```python
from build123d import *

# Parameters (mm, degrees)
SKETCH_5_R          = 36
CUT_EXTRUDE_1_DEPTH = 191
SKETCH_6_R          = 3
CUT_EXTRUDE_3_DEPTH = 225
SKETCH_7_R          = 2.7
CUT_EXTRUDE_4_DEPTH = 111


with BuildPart() as part:
    # 草图1 → 旋转6 (revolve)
    with BuildSketch(Plane(origin=(0, 0, 0), x_dir=(0, 0, -1), z_dir=(1, 0, 0)), mode=Mode.PRIVATE) as revolve_6_sk:
        with BuildLine():
            Line((3.317174788, 159.625816033), (43.317174788, 159.625816033))
            Line((43.317174788, 159.625816033), (73.317174788, 159.625816033))
            Line((73.317174788, 159.625816033), (73.317174788, 179.625816033))
            Line((73.317174788, 179.625816033), (81.317174788, 179.625816033))
            Line((81.317174788, 179.625816033), (81.317174788, 154.625816033))
            Line((81.317174788, 154.625816033), (73.317174788, 154.625816033))
            Line((73.317174788, 154.625816033), (53.317174788, 154.625816033))
            Line((53.317174788, 154.625816033), (53.317174788, 94.625816033))
            Line((53.317174788, 94.625816033), (43.317174788, 94.625816033))
            Line((43.317174788, 94.625816033), (43.317174788, 154.625816033))
            Line((43.317174788, 154.625816033), (3.317174788, 154.625816033))
            ThreePointArc((3.317174788, 154.625816033), (-39.109232083, 137.052222904), (-56.682825212, 94.625816033))
            Line((-56.682825212, 94.625816033), (-61.682825212, 94.625816033))
            ThreePointArc((-61.682825212, 94.625816033), (-42.644765989, 140.58775681), (3.317174788, 159.625816033))
        make_face()
    revolve(revolve_6_sk.sketch.rotate(Axis((0, 94.625816033, -43.317174788), (0, 0, -1)), 90), axis=Axis((0, 94.625816033, -43.317174788), (0, 0, -1)))

    # 草图5 → 切除-拉伸1 (cut)
    with BuildSketch(Plane(origin=(0, 0, 0), x_dir=(1, 0, 0), z_dir=(0, 1, 0))):
        with Locations(Location((0, 5.317174788, 0), (0, 0, 183.184738537))):
            Circle(SKETCH_5_R)
    extrude(amount=CUT_EXTRUDE_1_DEPTH, mode=Mode.SUBTRACT)

    # 草图6 → 切除-拉伸3 (cut)
    with BuildSketch(Plane.XY):
        with Locations((0, 169.625816033)):
            Circle(SKETCH_6_R)
        with Locations((0, 19.625816033)):
            Circle(SKETCH_6_R)
        with Locations((64.951905284, 132.125816033)):
            Circle(SKETCH_6_R)
        with Locations((64.951905284, 57.125816033)):
            Circle(SKETCH_6_R)
        with Locations((-64.951905284, 132.125816033)):
            Circle(SKETCH_6_R)
        with Locations((-64.951905284, 57.125816033)):
            Circle(SKETCH_6_R)
    extrude(amount=-CUT_EXTRUDE_3_DEPTH, mode=Mode.SUBTRACT)

    # 草图7 → 切除-拉伸4 (cut)
    with BuildSketch(Plane.XY):
        with Locations((0, 94.386174491)):
            Circle(SKETCH_7_R)
        with Locations((0, 114.625816033)):
            Circle(SKETCH_7_R)
        with Locations((0, 74.386174491)):
            Circle(SKETCH_7_R)
    extrude(amount=-CUT_EXTRUDE_4_DEPTH, mode=Mode.SUBTRACT)


solid = part.part
```
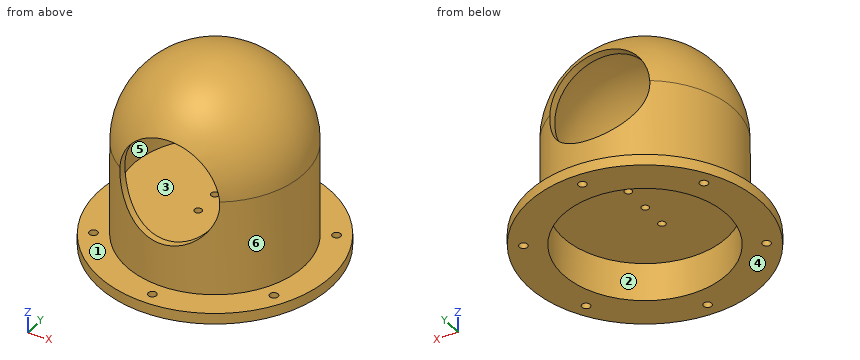
The model under review builds one solid part; all positions refer to its coordinate system, in mm. Face numbers are marked on the shaded views. A direction names the side the tool comes from. Round coordinates to 2 decimals unless told otherwise and drop trailing zeros. Loops run counter-clockwise (first coordinate to the right, second up) from the corner with the lowest first, then second, coordinate; pieces in that order, holes last. Notation, with made-up numbers: (30, 12.25) -> (62, 12.25) arc R16 cw to (62, 40.25) -> close; hole circle Ø7 at (89.25, 62). An arc over 180 degrees is marked (long way). Answer in a Markdown table with one row per item.
1) Draft analysis for pull direction Y (two halves, no side actions). For the marked faces 4, 5 and 6, state which applies: pulls with the +Y half, pulls with the -Y half, needs draft (parallel to the pull), parting line crosses it, or undercut.
Taken from the geometry:
| item | result |
|---|---|
| face 4 | needs draft |
| face 5 | undercut |
| face 6 | parting line crosses it |
2) Consider section A-A, the plane z = -14. Write out the cut boundary in (x, y), plus the area to 3 significant figures.
Taken from the geometry:
| item | result |
|---|---|
| outline | (-34.94, 39.81) -> (-34.94, 45.85) arc R60 cw to (-34.94, 143.4) -> (-34.94, 149.44) arc R65 ccw to start; (34.94, 39.81) arc R65 ccw to (34.94, 149.44) -> (34.94, 143.4) arc R60 cw to (34.94, 45.85) -> close |
| area | 1,220 mm² |
3) Tool access review of the marked faces 1, 2 and 3: name each direction out of +Z, -Z, +X, -X, +Y, -Y from which nothing blocks a thin tool from reaching the whole face with its end or side.
Taken from the geometry:
| item | result |
|---|---|
| face 1 | +Z |
| face 2 | -Z |
| face 3 | none |
4) Consider section C-C, the plane y = 68.5. Write out the cut boundary in (x, z).
Taken from the geometry:
| item | result |
|---|---|
| outline | (-80.89, -81.32) -> (-54.01, -81.32) -> (-54.01, -53.32) -> (54.01, -53.32) -> (54.01, -81.32) -> (80.89, -81.32) -> (80.89, -73.32) -> (59.52, -73.32) -> (59.52, -3.32) arc R59.52 ccw to (-59.52, -3.32) -> (-59.52, -73.32) -> (-80.89, -73.32) -> close; hole (-54.01, -43.32) -> (54.01, -43.32) -> (54.01, -3.32) arc R54.01 ccw to (-54.01, -3.32) -> close |
5) Consider section D-D, the plane z = -36.5. Write out the cut boundary in (x, y), plus the area to 3 significant figures.
Taken from the geometry:
| item | result |
|---|---|
| outline | (-17.99, 32.16) -> (-17.99, 37.39) arc R60 cw to (-17.99, 151.87) -> (-17.99, 157.09) arc R65 ccw to start; (17.99, 32.16) arc R65 ccw to (17.99, 157.09) -> (17.99, 151.87) arc R60 cw to (17.99, 37.39) -> close |
| area | 1,600 mm² |
6) Wall thickness on line 1 along Y through (x, z) = (0, -47); line 2 along Z through (x, y) = (34, 21.5); line 3 along X through (y, z) = (72, -19.5): over which ranges is each line inside the solid? List them lowest first.
Taken from the geometry:
| item | result |
|---|---|
| line 1 | y = 29.63 to 71.69, 77.09 to 91.69, 97.09 to 111.93, 117.33 to 159.63 |
| line 2 | z = -81.32 to -73.32 |
| line 3 | x = -60.93 to -55.57, 55.57 to 60.93 |
7) For pin 1 Ø4 at (y, z) = (138.5, 29.5) entering from +X; pin 2 Ø6 at (y, z) = (148.5, -44) entering from +X; pin 3 Ø2 at (y, z) = (93.5, 39) entering from -X, all flat-tipped, find the tip position at first contact; note any pin that passes through.
Taken from the geometry:
| item | result |
|---|---|
| pin 1 | stops at x = 37.92 |
| pin 2 | stops at x = 40.46 |
| pin 3 | stops at x = -50.17 |
8) Consider section B-B, the plane x = 22.5. Write out the cut boundary in (y, z), plus the area to 3 significant figures.
Taken from the geometry:
| item | result |
|---|---|
| outline | (12.66, -81.32) -> (39, -81.32) -> (39, -53.32) -> (150.25, -53.32) -> (150.25, -81.32) -> (176.59, -81.32) -> (176.59, -73.32) -> (155.61, -73.32) -> (155.61, -33.42) -> (150.25, -33.42) -> (150.25, -43.32) -> (39, -43.32) -> (39, -33.42) -> (33.64, -33.42) -> (33.64, -73.32) -> (12.66, -73.32) -> close; (39.51, 22.79) -> (45.51, 22.79) arc R55.62 cw to (143.74, 22.79) -> (149.74, 22.79) arc R60.98 ccw to start |
| area | 2,650 mm² |
